Autodesk Inventor part; units mm, degrees
ref_plane "YZ Plane" through (0, 0, 0) normal (1, 0, 0) x (0, 1, 0)
ref_plane "XZ Plane" through (0, 0, 0) normal (0, 1, 0) x (-1, 0, 0)
ref_plane "XY Plane" through (0, 0, 0) normal (0, 0, 1) x (1, 0, 0)
sketch "Sketch1" plane through (0, 0, 0) normal (0, 0, 1) x (1, 0, 0)
  line L0 (0, 0) -> (19, 0)
  line L1 (19, 0) -> (19, 339)
  line L2 (19, 339) -> (0, 339)
  line L3 (0, 339) -> (0, 0)
  dimension "d0" = 19
  dimension "d1" = 339
extrude "Extrusion1" add sketch "Sketch1" along normal blind 19
sketch "Sketch2" plane through (0, 0, 0) normal (0, -1, 0) x (1, 0, 0)
  line L0 (0, 0) -> (19, 0)
  line L1 (19, 0) -> (19, 19)
  line L2 (0, 19) -> (19, 19)
  line L3 (0, 0) -> (0, 19)
  line L4 (17.5, 17.5) -> (17.5, 1.5)
  line L5 (17.5, 1.5) -> (1.5, 1.5)
  line L6 (1.5, 1.5) -> (1.5, 17.5)
  line L7 (1.5, 17.5) -> (17.5, 17.5)
  dimension "d4" = 1.5
extrude "Extrusion2" cut sketch "Sketch2" against normal through all contours L4 L5 L6 L7
properties part number "C008" material "Aluminum 6061"
Geometry: final body of the model. Coordinates: model frame, mm. A direction names the side the tool comes from. Coordinates: 2 decimals unless noted, no trailing zeros. Loops run counter-clockwise (first coordinate to the right, second up) from the corner with the lowest first, then second, coordinate; pieces in that order, holes last. Notation, with made-up numbers: (21, 61) -> (42, 61) arc R14 ccw to (42, 75) -> close; hole circle Ø8 at (-28, 59). An arc over 180 degrees is marked (long way). Use a Markdown table: item, result. Add a question column.
(1) Section query A-A, the plane x = 9.75. Return loops of the section in (y, z).
(2) Line query: line 1 along X through (y, z) = (80.5, 15.75). Output: solid intervals per line, ascending.
(3) Section query C-C, the plane y = 164. Return loops of the section in (x, z), plus the area to 3 significant figures.
(4) Pin query (flat end, axial travel): pin 1 Ø3 at (y, z) = (130, 8.5) entering from -X. Return the tip coordinate at first contact, or that it passes through.
(5) Mould query, pull axis X, two halves, no side actions, for faces 3 (the flat face through (9, 167, 17.5)), 4 (the flat face through (19, 167, 9)), 5 (the flat face through (9, 0, 18)), 6 (the flat face through (10, 167, 1.5)). Classes: pulls with the +X half, pulls with the -X half, needs draft (parallel to the pull), parting line crosses it, or undercut.
(6) Section query B-B, the plane z = 9.25. Return loops of the section in (x, y), plus the area to 3 significant figures.
(7) Access query for faces 1 (the flat face through (0, 172, 9)), 2 (the flat face through (17.5, 167, 10)). Directions: +Z, -Z, +X, -X, +Y, -Y. A direction counts if a zero-diameter tool reaches every point of the face in a straight line with its end or side. Return the directions, or none.
Answer:
| question | item | result |
|---|---|---|
| 1 | outline | (0, 0) -> (339, 0) -> (339, 1.5) -> (0, 1.5) -> close; (0, 17.5) -> (339, 17.5) -> (339, 19) -> (0, 19) -> close |
| 2 | line 1 | x = 0 to 1.5, 17.5 to 19 |
| 3 | outline | (0, 0) -> (19, 0) -> (19, 19) -> (0, 19) -> close; hole (1.5, 1.5) -> (17.5, 1.5) -> (17.5, 17.5) -> (1.5, 17.5) -> close |
| 3 | area | 105 mm^2 |
| 4 | pin 1 | stops at x = 0 |
| 5 | face 3 | undercut |
| 5 | face 4 | pulls with the +X half |
| 5 | face 5 | needs draft |
| 5 | face 6 | undercut |
| 6 | outline | (0, 0) -> (1.5, 0) -> (1.5, 339) -> (0, 339) -> close; (17.5, 0) -> (19, 0) -> (19, 339) -> (17.5, 339) -> close |
| 6 | area | 1,020 mm^2 |
| 7 | face 1 | +Z, -Z, -X, +Y, -Y |
| 7 | face 2 | +Y, -Y |
